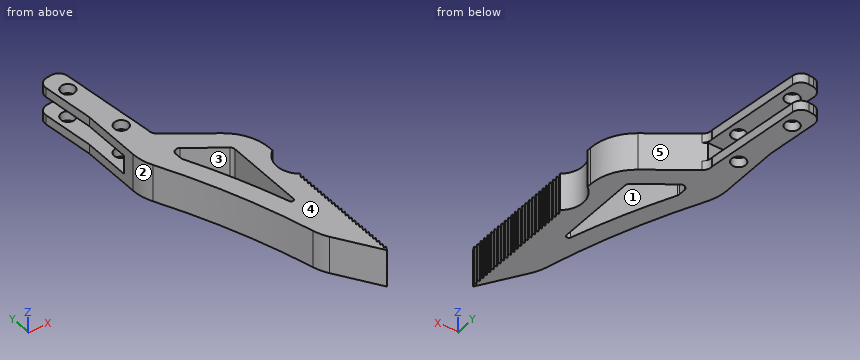
```python
from build123d import *

# Parameters (mm, degrees)
BOSS_EXTRUDE1_DEPTH     = 4
SKETCH2_W               = 20
SKETCH2_H               = 25
CUT_EXTRUDE1_DEPTH      = 2
CUT_EXTRUDE2_DEPTH      = 78.699873386
CUT_EXTRUDE2_DEPTH_BACK = 78.699873386
CUT_EXTRUDE3_DEPTH      = 78.699873386
LPATTERN3_START         = -4
LPATTERN3_DEPTH         = 8
CUT_EXTRUDE4_DEPTH      = 78.699873386
CUT_EXTRUDE5_DEPTH      = 78.699873386
FILLET1_R               = 10
FILLET2_R               = 2
FILLET3_R               = 1
FILLET4_R               = 0.5
SKETCH7_R               = 1.5
CUT_EXTRUDE6_DEPTH      = 78.443079806


# Read off the part's stored shape, not the designer's step: LPattern3
with BuildPart() as part:
    # Sketch1 → Boss-Extrude1 (new, symmetric)
    with BuildSketch(Plane.XY):
        Polygon((0, 0), (-20, 30.652242985), (-20, 60.782242985), (-21.435566599, 73.70273634), (-16.466146078, 74.25487734), (-14.000284373, 52.061445292), (-14.000284373, 50.661445292), (0, 40.6751395), align=None)
    extrude(amount=BOSS_EXTRUDE1_DEPTH, both=True)

    # Sketch2 → Cut-Extrude1 (cut, symmetric)
    with BuildSketch(Plane.XY):
        with Locations((-24.000284373, 63.161445292)):
            Rectangle(SKETCH2_W, SKETCH2_H)
    extrude(amount=CUT_EXTRUDE1_DEPTH, both=True, mode=Mode.SUBTRACT)

    # Sketch3 → Cut-Extrude2 (cut, two sides: drawn at the far end of the back side and taken through both)
    with BuildSketch(Plane.XY.offset(4).offset(-CUT_EXTRUDE2_DEPTH_BACK)):
        with BuildLine():
            Line((91.496624596, 103.297607947), (0, 34.6751395))
            ThreePointArc((0, 34.6751395), (-2, 30.6751395), (0, 26.6751395))
            Line((0, 26.6751395), (91.496624596, -41.947328947))
            Line((91.496624596, -41.947328947), (320.238186086, -41.947328947))
            Line((320.238186086, -41.947328947), (320.238186086, 103.297607947))
            Line((320.238186086, 103.297607947), (91.496624596, 103.297607947))
        make_face()
    extrude(amount=CUT_EXTRUDE2_DEPTH + CUT_EXTRUDE2_DEPTH_BACK, mode=Mode.SUBTRACT)

    # Sketch4 → Cut-Extrude3 (cut, symmetric)
    with BuildSketch(Plane.XY.offset(4)):
        Polygon((0, 26.6751395), (-0.5, 25.6751395), (0, 25.6751395), align=None)
    extrude(amount=CUT_EXTRUDE3_DEPTH, both=True, mode=Mode.SUBTRACT)

    # LPattern3 outline → LPattern3 (cut)
    with BuildSketch(Plane.XY.offset(LPATTERN3_START)):
        Polygon((0, 0), (0, 1.6126395), (-0.456500581, 0.699638337), align=None)
        Polygon((-0.5, 24.6726395), (0, 24.6726395), (0, 25.6726395), align=None)
        Polygon((-0.5, 23.6701395), (0, 23.6701395), (0, 24.6701395), align=None)
        Polygon((-0.5, 22.6676395), (0, 22.6676395), (0, 23.6676395), align=None)
        Polygon((-0.5, 21.6651395), (0, 21.6651395), (0, 22.6651395), align=None)
        Polygon((-0.5, 20.6626395), (0, 20.6626395), (0, 21.6626395), align=None)
        Polygon((-0.5, 19.6601395), (0, 19.6601395), (0, 20.6601395), align=None)
        Polygon((-0.5, 18.6576395), (0, 18.6576395), (0, 19.6576395), align=None)
        Polygon((-0.5, 17.6551395), (0, 17.6551395), (0, 18.6551395), align=None)
        Polygon((-0.5, 16.6526395), (0, 16.6526395), (0, 17.6526395), align=None)
        Polygon((-0.5, 15.6501395), (0, 15.6501395), (0, 16.6501395), align=None)
        Polygon((-0.5, 14.6476395), (0, 14.6476395), (0, 15.6476395), align=None)
        Polygon((-0.5, 13.6451395), (0, 13.6451395), (0, 14.6451395), align=None)
        Polygon((-0.5, 12.6426395), (0, 12.6426395), (0, 13.6426395), align=None)
        Polygon((-0.5, 11.6401395), (0, 11.6401395), (0, 12.6401395), align=None)
        Polygon((-0.5, 10.6376395), (0, 10.6376395), (0, 11.6376395), align=None)
        Polygon((-0.5, 9.6351395), (0, 9.6351395), (0, 10.6351395), align=None)
        Polygon((-0.5, 8.6326395), (0, 8.6326395), (0, 9.6326395), align=None)
        Polygon((-0.5, 7.6301395), (0, 7.6301395), (0, 8.6301395), align=None)
        Polygon((-0.5, 6.6276395), (0, 6.6276395), (0, 7.6276395), align=None)
        Polygon((-0.5, 5.6251395), (0, 5.6251395), (0, 6.6251395), align=None)
        Polygon((-0.5, 4.6226395), (0, 4.6226395), (0, 5.6226395), align=None)
        Polygon((-0.5, 3.6201395), (0, 3.6201395), (0, 4.6201395), align=None)
        Polygon((-0.5, 2.6176395), (0, 2.6176395), (0, 3.6176395), align=None)
        Polygon((-0.5, 1.6151395), (0, 1.6151395), (0, 2.6151395), align=None)
    extrude(amount=LPATTERN3_DEPTH, mode=Mode.SUBTRACT)

    # Sketch5 → Cut-Extrude4 (cut, through all)
    with BuildSketch(Plane.XY.offset(4)):
        with BuildLine():
            Line((-20, 45.652242985), (-20, 30.652242985))
            Line((-20, 30.652242985), (-7.147540984, 10.954408149))
            ThreePointArc((-7.147540984, 10.954408149), (-12.567364929, 28.676109238), (-20, 45.652242985))
        make_face()
    extrude(amount=-CUT_EXTRUDE4_DEPTH, mode=Mode.SUBTRACT)

    # Sketch6 → Cut-Extrude5 (cut, through all)
    with BuildSketch(Plane.XY.offset(4)):
        with BuildLine():
            Line((-14.004117633, 45.750871885), (-5, 39.328297195))
            Line((-5, 39.328297195), (-5, 18.390871885))
            ThreePointArc((-5, 18.390871885), (-9.031897039, 30.419496018), (-14.004117633, 42.090871885))
            Line((-14.004117633, 42.090871885), (-14.004117633, 45.750871885))
        make_face()
    extrude(amount=-CUT_EXTRUDE5_DEPTH, mode=Mode.SUBTRACT)

    # Fillet1
    fillet1_edges = [part.edges().sort_by_distance(p)[0] for p in [
        (-20, 45.652242985, 0),
        (-7.147540984, 10.954408149, 0),
        (0, 40.6751395, 0),
    ]]
    fillet(fillet1_edges, radius=FILLET1_R)

    # Fillet2
    fillet2_edges = [part.edges().sort_by_distance(p)[0] for p in [
        (-14.000284373, 50.661445292, -3),
        (-16.466146078, 74.25487734, -3),
        (-21.435566599, 73.70273634, -3),
        (-14.000284373, 50.661445292, 3),
        (-16.466146078, 74.25487734, 3),
        (-21.435566599, 73.70273634, 3),
    ]]
    fillet(fillet2_edges, radius=FILLET2_R)

    # Fillet3
    fillet3_edges = [part.edges().sort_by_distance(p)[0] for p in [
        (-14.004117633, 42.090871885, 0),
        (-14.004117633, 45.750871885, 0),
        (-5, 39.328297195, 0),
    ]]
    fillet(fillet3_edges, radius=FILLET3_R)

    # Fillet4
    fillet4_edges = [part.edges().sort_by_distance(p)[0] for p in [
        (-5, 18.390871885, 0),
    ]]
    fillet(fillet4_edges, radius=FILLET4_R)

    # Sketch7 → Cut-Extrude6 (cut, through all)
    with BuildSketch(Plane.XY.offset(4)):
        with Locations((-18.416383851, 69.168407775)):
            Circle(SKETCH7_R)
        with Locations((-16.915664614, 55.661522799)):
            Circle(SKETCH7_R)
    extrude(amount=-CUT_EXTRUDE6_DEPTH, mode=Mode.SUBTRACT)


solid = part.part
```
Verification items for the finished model (mm, model axes). Face numbers are marked on the shaded views. A direction names the side the tool comes from. Give positions to 0.01 mm unless a question says otherwise; leave off trailing zeros. Loops run counter-clockwise (first coordinate to the right, second up) from the corner with the lowest first, then second, coordinate; pieces in that order, holes last. Notation, with made-up numbers: M 34.25,31 L 58.25,31 A19 cw 58.25,38 Z; hole C 16,12.5 d11. An arc over 180 degrees is marked long. One line per question, with ' | ' between items.
Item 1: Thickness scan on line 1 (Z direction, x = -20, y = 64); line 2 (X direction, y = 31.5, z = 1.25); line 3 (X direction, y = 70, z = 2.5). Record the ranges inside material, lowest first. Write a range as [from, to].
Completed:
line 1: z = [-4, -2], [2, 4] | line 2: x = [-13.64, -9.45], [-5, -1.93] | line 3: x = [-21.02, -19.66], [-17.17, -15.99]
Item 2: Section check C-C, the plane z = -2.75. State how many separate pieces and enclosed holes the cut face has, plus the area to 3 significant figures.
Completed:
separate pieces: 1 | enclosed holes: 3 | area: 499 mm^2
Item 3: Tool access check on the marked faces 1 and 2. Record the directions out of +Z, -Z, +X, -X, +Y, -Y that give a thin tool (end or side, any length) a straight path to the whole face; none if there is none.
Completed:
face 1: +Z, -Z | face 2: +Z, -Z, -X, -Y
Item 4: Depth check by flat-ended pin: P1, Ø2, axis at x = -15.5, z = 2.5, coming from the +Y side; P2, Ø1.6, axis at y = 43.5, z = -0.5, coming from the +X side; P3, Ø2, axis at y = 64, z = 1.5, coming from the -X side. Enter the tip coordinate at first touch or a pass-through.
Completed:
P1: stops at y = 73.04 | P2: stops at x = -3.03 | P3: stops at x = -20.45
Item 5: Section check D-D, the plane y = 46. Record the cut outline in (x, z).
Completed:
outline: M -19.8,-4 L -7.47,-4 L -7.47,4 L -19.8,4 Z
Item 6: Section check B-B, the plane y = 67. Record the cut outline in (x, z).
Completed:
outline: M -20.69,-4 L -15.66,-4 L -15.66,-2 L -20.69,-2 Z; M -20.69,2 L -15.66,2 L -15.66,4 L -20.69,4 Z
Item 7: Draft check along X on the marked faces 3, 4 and 5. Enter one of: +X half, -X half, draft (parallel to the pull), parting line (faces both ways), or undercut.
Completed:
face 3: undercut | face 4: draft | face 5: +X half
Item 8: Section check A-A, the plane y = 33. Record the cut outline in (x, z).
Completed:
outline: M -14.24,-4 L -10.04,-4 L -10.04,4 L -14.24,4 Z; M -5,-4 L -1.43,-4 L -1.43,4 L -5,4 Z
